Geometry: final body of the model. Coordinates: model frame, mm. Give positions to 0.01 mm unless a question says otherwise; leave off trailing zeros. Write each loop counter-clockwise with the first axis right and the second up, starting at its lowest first coordinate (ties: lowest second). Pieces come first, ordered by that corner, then holes. Notation, with made-up numbers: (-14.75, 3) - (31.25, 3) arc R20 cw to (31.25, 35) - close; hole circle Ø2 at (66, -12.75). An arc over 180 degrees is marked (long way). Return JSON: item names as keys, results as strings.
Autodesk Inventor part; units mm, degrees
ref_plane "YZ Plane" through (0, 0, 0) normal (1, 0, 0) x (0, 1, 0)
ref_plane "XZ Plane" through (0, 0, 0) normal (0, 1, 0) x (-1, 0, 0)
ref_plane "XY Plane" through (0, 0, 0) normal (0, 0, 1) x (1, 0, 0)
sketch "Sketch1" plane through (0, 0, 0) normal (1, 0, 0) x (0, 1, 0)
  line L0 (11.1125, 11.1125) -> (-11.1125, 11.1125)
  line L1 (-11.1125, 11.1125) -> (-11.1125, -11.1125)
  line L2 (-11.1125, -11.1125) -> (11.1125, -11.1125)
  line L3 (11.1125, -11.1125) -> (11.1125, 11.1125)
  line L4 (12.7, 12.7) -> (-12.7, 12.7)
  line L5 (-12.7, 12.7) -> (-12.7, -12.7)
  line L6 (-12.7, -12.7) -> (12.7, -12.7)
  line L7 (12.7, -12.7) -> (12.7, 12.7)
  line L8 (0, 11.1125) -> (0, 12.7) construction
  line L9 (11.1125, 0) -> (12.7, 0) construction
  line L10 (11.1125, 0) -> (0, 0) construction
  line L11 (0, 0) -> (0, 11.1125) construction
  dimension "d0" = 25.4
  dimension "d1" = 1.5875
extrude "Extrusion1" add sketch "Sketch1" along normal blind 457.2
sketch "Sketch2" plane through (0, -12.7, 12.7) normal (0, 0, 1) x (1, 0, 0)
  line L0 (0, 12.7) -> (457.2, 12.7) construction
  line L1 (457.2, 1.5875) -> (457.2, 23.8125) construction
  circle A0 centre (450.85, 12.7) radius 1.5875
  circle A1 centre (431.8, 12.7) radius 1.5875
  line L2 (228.6, 12.7) -> (228.6, 1.5875) construction
  circle A2 centre (6.35, 12.7) radius 1.5875
  circle A3 centre (25.4, 12.7) radius 1.5875
  dimension "d4" = 6.35
  dimension "d5" = 19.05
  dimension "d6" = 3.175
extrude "Extrusion2" cut sketch "Sketch2" against normal up to next
sketch "Sketch3" plane through (0, 12.7, 12.7) normal (0, 1, 0) x (1, 0, 0)
  line L0 (0, 0) -> (457.2, 0) construction
  line L1 (228.6, 0) -> (228.6, 42.8948) construction
  line L2 (361.95, 0) -> (361.95, 36.7793) construction
  circle A0 centre (361.95, 6.35) radius 1.5875
  circle A1 centre (361.95, 19.05) radius 1.5875
  circle A2 centre (95.25, 6.35) radius 1.5875
  circle A3 centre (95.25, 19.05) radius 1.5875
  circle A4 centre (228.6, 19.05) radius 1.5875
  circle A5 centre (228.6, 6.35) radius 1.5875
  line L3 (361.95, 19.05) -> (228.6, 19.05) construction
  line L4 (0, 23.8125) -> (457.2, 23.8125) construction
  line L5 (361.95, 6.35) -> (228.6, 6.35) construction
  point P0 (0, 12.7)
  dimension "d9" = 3.175
  dimension "d10" = 6.35
  dimension "d11" = 12.7
  dimension "d15" = 266.7
extrude "Extrusion3" cut sketch "Sketch3" against normal up to next
properties part number "Cross Brace"
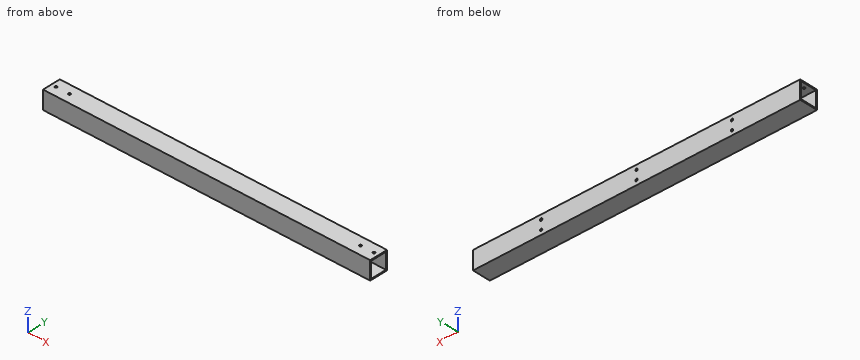
Q1. Material intervals for probe 1 along X at (y, z) = (11.8, -6.35); probe 2 along Z at (x, y) = (361.95, 12.15); probe 3 along Z at (x, y) = (38.5, 0.75), sorted ascending. Write a range as [from, to].
Answer key:
{"probe 1": "x = [0, 93.66], [96.84, 227.01], [230.19, 360.36], [363.54, 457.2]", "probe 2": "z = [-12.7, -7.94], [-4.76, 4.76], [7.94, 12.7]", "probe 3": "z = [-12.7, -11.11], [11.11, 12.7]"}
Q2. Pin query (flat end, axial travel): P1, Ø2.5, axis at x = 361.95, z = 6.35, coming from the +Y side; P2, Ø3, axis at x = 25.4, y = 0, coming from the +Z side. Return the tip coordinate at first contact, or that it passes through.
Answer key:
{"P1": "stops at y = -11.11", "P2": "stops at z = -11.11"}
Q3. Section query A-A, the plane y = 6.75. Return the cut outline in (x, z).
Answer key:
{"outline": "(0, -12.7) - (457.2, -12.7) - (457.2, -11.11) - (0, -11.11) - close; (0, 11.11) - (457.2, 11.11) - (457.2, 12.7) - (0, 12.7) - close"}
Q4. Section query C-C, the plane x = 271. Return the cut outline in (y, z), plus the area to 3 significant figures.
Answer key:
{"outline": "(-12.7, -12.7) - (12.7, -12.7) - (12.7, 12.7) - (-12.7, 12.7) - close; hole (-11.11, -11.11) - (11.11, -11.11) - (11.11, 11.11) - (-11.11, 11.11) - close", "area": "151 mm^2"}
